Work out the finished part from the listing and answer in its coordinate system (mm). Round coordinates to 2 decimals unless told otherwise and drop trailing zeros. Write each loop counter-clockwise with the first axis right and the second up, starting at its lowest first coordinate (ties: lowest second). Pieces come first, ordered by that corner, then holes. Notation, with made-up numbers: M 27.25,4.5 L 72.25,4.5 A13 cw 72.25,16.5 Z; hole C 85,56 d1. An arc over 180 degrees is marked long. One line per item, written item: value. Start each with the question number.
Q1. Given pin 1 Ø0.6 at (x, z) = (-8.5, -91) entering from +Y; pin 2 Ø3 at (y, z) = (8, -120.5) entering from +X; pin 3 Ø5 at (y, z) = (3, -89) entering from +X, each flat-ended and moving along its own axis, determine where each tip first touches the part or whether it passes through.
Q2. Find section A-A (z = -129). Write down the section's boundary in (x, y) (1 decimal).
Q3. Find section B-B (x = -5.25). Write down the section's boundary in (y, z) (3 decimals), and give its area (3 significant figures).
Q4. Consider probe 1 along Y at (x, z) = (-0.5, -36); probe 2 along X at (y, z) = (4.25, -47) (3 decimals); probe 3 along Y at (x, z) = (-5.5, -89). Determine where each line is inside the solid, lowest interval first.
Q5. Find section C-C (y = 2.5). Write down the section's boundary in (x, z) (3 decimals).
from build123d import *

# Parameters (mm, degrees)
EXTRUDE_THIN1_DEPTH = 142.875
FILLET1_R           = 0.889


with BuildPart() as part:
    # Sketch1 → Extrude-Thin1 (new body)
    with BuildSketch(Plane.XY):
        with BuildLine():
            Line((-0.396875, 0), (-9.525, 0))
            Line((-9.525, 0), (-9.525, 5.55625))
            Line((-9.525, 5.55625), (-7.9375, 5.55625))
            Line((-7.9375, 5.55625), (-7.9375, 7.14375))
            ThreePointArc((-7.9375, 7.14375), (-6.310112053, 11.072612053), (-2.38125, 12.7))
            Line((-2.38125, 12.7), (-2.38125, 14.2875))
            Line((-2.38125, 14.2875), (0, 14.2875))
            Line((0, 14.2875), (-0.396875, 11.1125))
            Line((-0.396875, 11.1125), (-1.279010032, 11.222766879))
            Line((-1.279010032, 11.222766879), (-1.007043392, 13.3985))
            Line((-1.007043392, 13.3985), (-1.49225, 13.3985))
            Line((-1.49225, 13.3985), (-1.49225, 11.725551126))
            ThreePointArc((-1.49225, 11.725551126), (-5.350596503, 10.744611551), (-7.0485, 7.14375))
            Line((-7.0485, 7.14375), (-7.0485, 4.66725))
            Line((-7.0485, 4.66725), (-8.636, 4.66725))
            Line((-8.636, 4.66725), (-8.636, 0.889))
            Line((-8.636, 0.889), (-0.396875, 0.889))
            Line((-0.396875, 0.889), (-0.396875, 0))
        make_face()
    extrude(amount=-EXTRUDE_THIN1_DEPTH)

    # Fillet1
    fillet1_edges = [part.edges().sort_by_distance(p)[0] for p in [
        (-1.49225, 11.725551126, -71.4375),
        (-7.0485, 4.66725, -71.4375),
        (-9.525, 0, -71.4375),
        (-9.525, 5.55625, -71.4375),
        (-2.38125, 14.2875, -71.4375),
    ]]
    fillet(fillet1_edges, radius=FILLET1_R)


solid = part.part
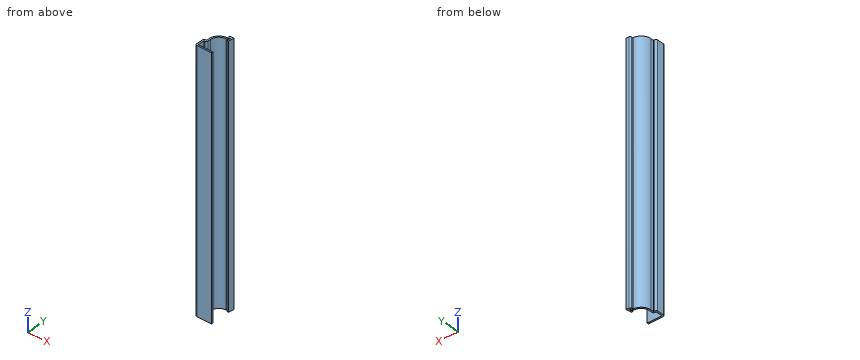
The answers:
1. pin 1: y = 5.56
1. pin 2: x = -6.41
1. pin 3: x = -0.4
2. outline: M -9.5,0.9 A0.9 ccw -8.6,0 L -0.4,0 L -0.4,0.9 L -8.6,0.9 L -8.6,4.7 L -7.9,4.7 A0.9 ccw -7,5.6 L -7,7.1 A4.7 cw -2.4,11.8 A0.9 ccw -1.5,12.7 L -1.5,13.4 L -1,13.4 L -1.3,11.2 L -0.4,11.1 L 0,14.3 L -1.5,14.3 A0.9 ccw -2.4,13.4 L -2.4,12.7 A5.6 ccw -7.9,7.1 L -7.9,5.6 L -8.6,5.6 A0.9 ccw -9.5,4.7 Z
3. outline: M 0,-142.875 L 0.889,-142.875 L 0.889,0 L 0,0 Z; M 10.825,-142.875 L 11.902,-142.875 L 11.902,0 L 10.825,0 Z
3. area: 281 mm2
4. probe 1: 0 to 0.89, 11.13 to 14.29
4. probe 2: -9.525 to -8.636
4. probe 3: 0 to 0.89, 10.62 to 11.74
5. outline: M -9.525,-142.875 L -8.636,-142.875 L -8.636,0 L -9.525,0 Z
